```python
from build123d import *

# Parameters (mm, degrees)
BOSS_EXTRUDE1_DEPTH = 3.3
SKETCH2_W           = 2
SKETCH2_H           = 10.9
BOSS_EXTRUDE2_DEPTH = 0.9
BOSS_EXTRUDE3_DEPTH = 1.7


with BuildPart() as part:
    # Sketch1 → Boss-Extrude1 (new body)
    with BuildSketch(Plane.XY):
        with BuildLine():
            add(Edge.make_bspline(
                [(53.263961031, 6.363961031), (50.163311673, 10.524172065), (45.36862919, 13.803956999), (39.822404925, 16.35)],
                knots=[0, 0, 0, 0, 0.272957657, 0.272957657, 0.272957657, 0.272957657], degree=3))
            ThreePointArc((53.263961031, 6.363961031), (53.678515614, 5.92044982), (54.062227307, 5.45))
            Line((54.062227307, 5.45), (55.8, 5.45))
            Line((55.8, 5.45), (55.8, 14.85))
            Line((55.8, 14.85), (63.1, 14.85))
            Line((63.1, 14.85), (63.1, -14.85))
            Line((63.1, -14.85), (55.8, -14.85))
            Line((55.8, -14.85), (55.8, -5.45))
            Line((55.8, -5.45), (54.062227307, -5.45))
            ThreePointArc((54.062227307, -5.45), (53.678515614, -5.92044982), (53.263961031, -6.363961031))
            add(Edge.make_bspline(
                [(39.822404925, -16.35), (45.36862919, -13.803956999), (50.163311673, -10.524172065), (53.263961031, -6.363961031)],
                knots=[0.727042343, 0.727042343, 0.727042343, 0.727042343, 1, 1, 1, 1], degree=3))
            Line((39.822404925, -16.35), (64.6, -16.35))
            Line((64.6, -16.35), (64.6, 16.35))
            Line((64.6, 16.35), (39.822404925, 16.35))
        make_face()
    extrude(amount=-BOSS_EXTRUDE1_DEPTH)

    # Sketch2 → Boss-Extrude2 (add)
    with BuildSketch(Plane(origin=(0, 0, 0), x_dir=(-1, 0, 0), z_dir=(0, 0, -1))):
        Polygon((-61.1, -5.45), (-63.1, -5.45), (-63.1, -14.85), (-55.8, -14.85), (-55.8, -5.45), align=None)
        Polygon((-55.8, 5.45), (-55.8, 14.85), (-63.1, 14.85), (-63.1, 5.45), (-61.1, 5.45), align=None)
        with Locations((-62.1, 0)):
            Rectangle(SKETCH2_W, SKETCH2_H)
    extrude(amount=BOSS_EXTRUDE2_DEPTH)

    # Sketch3 → Boss-Extrude3 (add)
    with BuildSketch(Plane.XY.offset(-3.3)):
        with BuildLine():
            Line((54.062227307, 5.45), (55.8, 5.45))
            Line((55.8, 5.45), (55.8, 14.85))
            Line((55.8, 14.85), (63.1, 14.85))
            Line((63.1, 14.85), (63.1, -14.85))
            Line((63.1, -14.85), (55.8, -14.85))
            Line((55.8, -14.85), (55.8, -5.45))
            Line((55.8, -5.45), (54.062227307, -5.45))
            ThreePointArc((54.062227307, -5.45), (53.678515614, -5.92044982), (53.263961031, -6.363961031))
            add(Edge.make_bspline(
                [(53.263961031, -6.363961031), (50.163311673, -10.524172065), (45.36862919, -13.803956999), (39.822404925, -16.35)],
                knots=[0.727042343, 0.727042343, 0.727042343, 0.727042343, 1, 1, 1, 1], degree=3))
            Line((39.822404925, -16.35), (64.6, -16.35))
            Line((64.6, -16.35), (64.6, -15.05))
            Line((64.6, -15.05), (64.6, 15.05))
            Line((64.6, 15.05), (64.6, 16.35))
            Line((64.6, 16.35), (39.822404925, 16.35))
            add(Edge.make_bspline(
                [(39.822404925, 16.35), (45.36862919, 13.803956999), (50.163311673, 10.524172065), (53.263961031, 6.363961031)],
                knots=[0, 0, 0, 0, 0.272957657, 0.272957657, 0.272957657, 0.272957657], degree=3))
            ThreePointArc((53.263961031, 6.363961031), (53.678515614, 5.92044982), (54.062227307, 5.45))
        make_face()
    extrude(amount=-BOSS_EXTRUDE3_DEPTH)


solid = part.part
```
Model file for the job. Use its own axes, mm. A direction names the side the tool comes from. Round coordinates to 2 decimals unless told otherwise and drop trailing zeros. Write each loop counter-clockwise with the first axis right and the second up, starting at its lowest first coordinate (ties: lowest second). Pieces come first, ordered by that corner, then holes. Notation, with made-up numbers: M 45.5,89 L 68.5,89 A19 cw 68.5,96 Z; hole C 81,17.25 d7. An arc over 180 degrees is marked long. Put each result on its own line as item: value.
Item 1: Cut at B-B (y = 1.5). List the corners of the cut face in (x, z), and give its area (3 significant figures).
Responses:
outline: M 61.1,-0.9 L 63.1,-0.9 L 63.1,-5 L 64.6,-5 L 64.6,0 L 61.1,0 Z
area: 9.30 mm²
Item 2: Tool access for faces 1 (the flat face through (55.8, -10, -3)), 2 (the flat face through (64.6, 0, -2)), 3 (the cylindrical face through (53.67, 5.93, -2.46)): list every direction of +Z, -Z, +X, -X, +Y, -Y with a clear straight run to the whole face (end or side of a thin tool).
Responses:
face 1: -Z
face 2: +Z, -Z, +X, +Y, -Y
face 3: +Z, -Z, -X
Item 3: Cut at C-C (x = 62.75). List the corners of the cut face in (y, z), and give its area (3 significant figures).
Responses:
outline: M -16.35,-5 L -14.85,-5 L -14.85,-0.9 L 14.85,-0.9 L 14.85,-5 L 16.35,-5 L 16.35,0 L -16.35,0 Z
area: 41.7 mm²
Item 4: Cut at A-A (x = 60). List the corners of the cut face in (y, z).
Responses:
outline: M -16.35,-5 L -14.85,-5 L -14.85,-0.9 L -5.45,-0.9 L -5.45,0 L -16.35,0 Z; M 5.45,-0.9 L 14.85,-0.9 L 14.85,-5 L 16.35,-5 L 16.35,0 L 5.45,0 Z
Item 5: Flat gauge pins, fed straight in: P1, Ø3.5, axis at x = 60.5, y = 7, coming from the -Z side; P2, Ø0.7, axis at y = 0, z = -0.5, coming from the -X side; P3, Ø1.5, axis at y = -1, z = -3.5, coming from the -X side. Where does each tip first touch, or does it go through?
Responses:
P1: z = -0.9
P2: x = 61.1
P3: x = 63.1
Item 6: Mould opens along X. For faces 4 (the cylindrical face through (53.684, -5.914, -2.465)), 5 (the flat face through (60, -14.85, -3)), 6 (the flat face through (55, 5.45, -1)) say: +X half, -X half, draft (parallel to the pull), parting line (faces both ways), or undercut.
Responses:
face 4: -X half
face 5: undercut
face 6: draft
Item 7: Probe L1, parallel to Y at x = 54.25, z = -0.55; L2, parallel to Y at x = 58.25, z = -2; L3, parallel to Z at x = 60, y = 13. List the from-to ranges inside material, lowest first. Write a range as from..to.
Responses:
L1: -16.35..-5.45, 5.45..16.35
L2: -16.35..-14.85, 14.85..16.35
L3: -0.9..0
